Print and shaded views of the part. All mm, measured from the part's lowest x, y and z. Give positions to 0.01 mm unless a question says otherwise; leave off trailing zeros. Write each loop counter-clockwise with the first axis right and the second up, starting at its lowest first coordinate (ties: lowest second). Pieces come first, ordered by that corner, then holes.
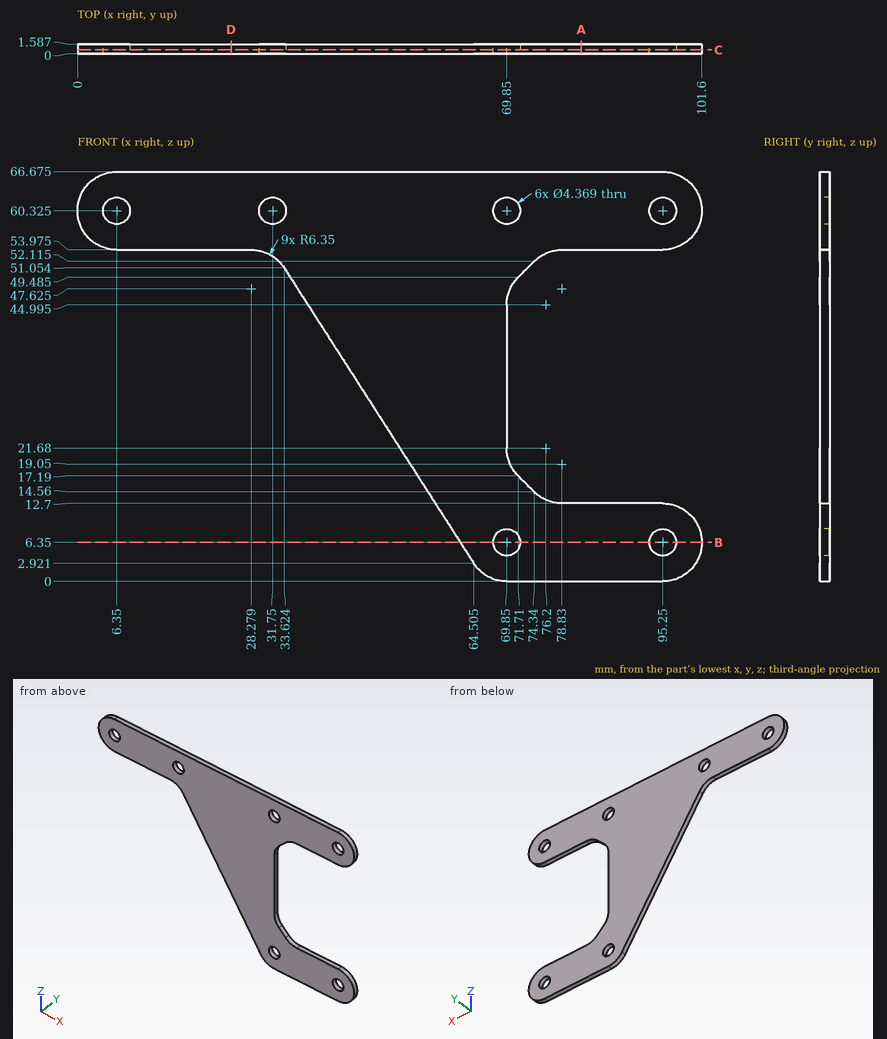
1. Saw through at A-A on x = 82. Give the cut face in (y, z) (1 decimal).
2. Saw through at B-B on z = 6.35. Give the cut face in (x, y) (1 decimal).
3. Drop flat-ended pins along their axis: pin 1 (6 mm diameter, centred on x = 46, z = 49, fed in from -Y); pin 2 (0.5 mm diameter, centred on x = 12.5, y = 1, fed in from -Z) (1 decimal). Give the stop position or say it passes through.
4. Saw through at C-C on y = 0.65. Count the separate pieces of the cut face and the enclosed holes in it, plus the area to 3 significant figures.
5. Saw through at D-D on x = 25. Give the cut face in (y, z) (1 decimal).
6. Drill centre lines: line 1 along X through (y, z) = (1.2, 60.5); line 2 along Z through (x, y) = (68, 1.55) (1 decimal); line 3 along Z through (x, y) = (6.5, 0.4) (1 decimal). Where is each one in solid material? Low to high.
Outcome:
1. outline: (0, 0) - (1.6, 0) - (1.6, 12.7) - (0, 12.7) - close; (0, 54) - (1.6, 54) - (1.6, 66.7) - (0, 66.7) - close
2. outline: (62.3, 0) - (67.7, 0) - (67.7, 1.6) - (62.3, 1.6) - close; (72, 0) - (93.1, 0) - (93.1, 1.6) - (72, 1.6) - close; (97.4, 0) - (101.6, 0) - (101.6, 1.6) - (97.4, 1.6) - close
3. pin 1: stops at y = 0
3. pin 2: stops at z = 54
4. separate pieces: 1
4. enclosed holes: 6
4. area: 2,720 mm2
5. outline: (0, 54) - (1.6, 54) - (1.6, 66.7) - (0, 66.7) - close
6. line 1: x = 0 to 4.17, 8.53 to 29.57, 33.93 to 67.67, 72.03 to 93.07, 97.43 to 101.6
6. line 2: z = 0.3 to 5.2, 7.5 to 59.2, 61.5 to 66.7
6. line 3: z = 54 to 58.1, 62.5 to 66.7
